from build123d import *

# Parameters (mm, degrees)
F0_W     = 50
F0_H     = 75
F1_DEPTH = 4
F2_W     = 42
F2_H     = 67
F3_DEPTH = 4
F4_R     = 3
F5_R     = 2
F6_DEPTH = 25


with BuildPart() as f1:
    # F0 (on Top) → F1 (new body)
    with BuildSketch(Plane.XY):
        with Locations((25, -37.5)):
            Rectangle(F0_W, F0_H)
    extrude(amount=F1_DEPTH)

    # F2 (on face) → F3 (join)
    with BuildSketch(Plane.XY.offset(4)):
        with Locations((25, -37.5)):
            Rectangle(F2_W, F2_H)
    extrude(amount=F3_DEPTH)

    # F4
    f4_edges = [f1.edges().sort_by_distance(p)[0] for p in [
        (50, 0, 2),
        (4, -4, 6),
        (0, 0, 2),
        (46, -4, 6),
        (46, -71, 6),
        (50, -75, 2),
        (4, -71, 6),
        (0, -75, 2),
    ]]
    fillet(f4_edges, radius=F4_R)

    # F5 (on face) → F6 (cut)
    with BuildSketch(Plane.XY.offset(8)):
        with Locations((25, -51)):
            Circle(F5_R)
        with Locations((25, -24)):
            Circle(F5_R)
    extrude(amount=-F6_DEPTH, mode=Mode.SUBTRACT)


solid = f1.part
Work out the finished part from the listing and answer in its coordinate system (mm). A direction names the side the tool comes from. Coordinates: 2 decimals unless noted, no trailing zeros. Write each loop counter-clockwise with the first axis right and the second up, starting at its lowest first coordinate (ties: lowest second). Pieces come first, ordered by that corner, then holes.
1. The part is cut by section B-B, the plane x = 25. Write down the section's boundary in (y, z), and give its area (3 significant figures).
Results list:
outline: (-75, 0) - (-53, 0) - (-53, 8) - (-71, 8) - (-71, 4) - (-75, 4) - close; (-49, 0) - (-26, 0) - (-26, 8) - (-49, 8) - close; (-22, 0) - (0, 0) - (0, 4) - (-4, 4) - (-4, 8) - (-22, 8) - close
area: 504 mm2
2. For a pull along Y with two mould halves and no side action, classify faces 6 (the flat face through (25, -37, 8)), 7 (the flat face through (25, -71, 6)), 8 (the cylindrical face through (25, -53, 4)) as +Y half, -Y half, draft (parallel to the pull), parting line (faces both ways), or undercut.
Results list:
face 6: draft
face 7: -Y half
face 8: undercut
3. Flat-ended cylindrical pins translate along their axes: pin 1 (1.2 mm diameter, centred on y = -35.5, z = 6.5, fed in from +X); pin 2 (1 mm diameter, centred on x = 22.5, z = 5, fed in from +Y); pin 3 (1.5 mm diameter, centred on y = -41.5, z = 7, fed in from -X); pin 4 (3 mm diameter, centred on x = 30, z = 5, fed in from +Y). Find the tip coordinate at first contact, or state that the pin passes through.
Results list:
pin 1: stops at x = 46
pin 2: stops at y = -4
pin 3: stops at x = 4
pin 4: stops at y = 0
4. The part is cut by section D-D, the plane x = 37. Write down the section's boundary in (y, z).
Results list:
outline: (-75, 0) - (0, 0) - (0, 4) - (-4, 4) - (-4, 8) - (-71, 8) - (-71, 4) - (-75, 4) - close
5. For faces 1 (the flat face through (4, -38, 6)), 2 (the cylindrical face through (45.14, -4.9, 6.03)), 3 (the flat face through (46, -38, 6)), 4 (the cylindrical face through (4.9, -70.14, 6.03)), 5 (the cylindrical face through (4.9, -4.86, 6.03)), determine the directions among +Z, -Z, +X, -X, +Y, -Y from which every point of the face is accessible in a straight line to the end or side of a thin tool.
Results list:
face 1: +Z, -X, +Y, -Y
face 2: +Z, +X, +Y
face 3: +Z, +X, +Y, -Y
face 4: +Z, -X, -Y
face 5: +Z, -X, +Y
6. The part is cut by section C-C, the plane z = 5.75. Write down the section's boundary in (x, y).
Results list:
outline: (4, -68) arc R3 ccw to (7, -71) - (43, -71) arc R3 ccw to (46, -68) - (46, -7) arc R3 ccw to (43, -4) - (7, -4) arc R3 ccw to (4, -7) - close; hole circle Ø4 at (25, -51); hole circle Ø4 at (25, -24)
7. Consider line 1 along Y through (x, z) = (25, 6.25); line 2 along Y through (x, z) = (25, 2.75); line 3 along Y through (x, z) = (9, 5). Determine where each line is inside the solid, lowest interval first.
Results list:
line 1: y = -71 to -53, -49 to -26, -22 to -4
line 2: y = -75 to -53, -49 to -26, -22 to 0
line 3: y = -71 to -4
8. The part is cut by section A-A, the plane y = -51. Write down the section's boundary in (x, z).
Results list:
outline: (0, 0) - (23, 0) - (23, 8) - (4, 8) - (4, 4) - (0, 4) - close; (27, 0) - (50, 0) - (50, 4) - (46, 4) - (46, 8) - (27, 8) - close
